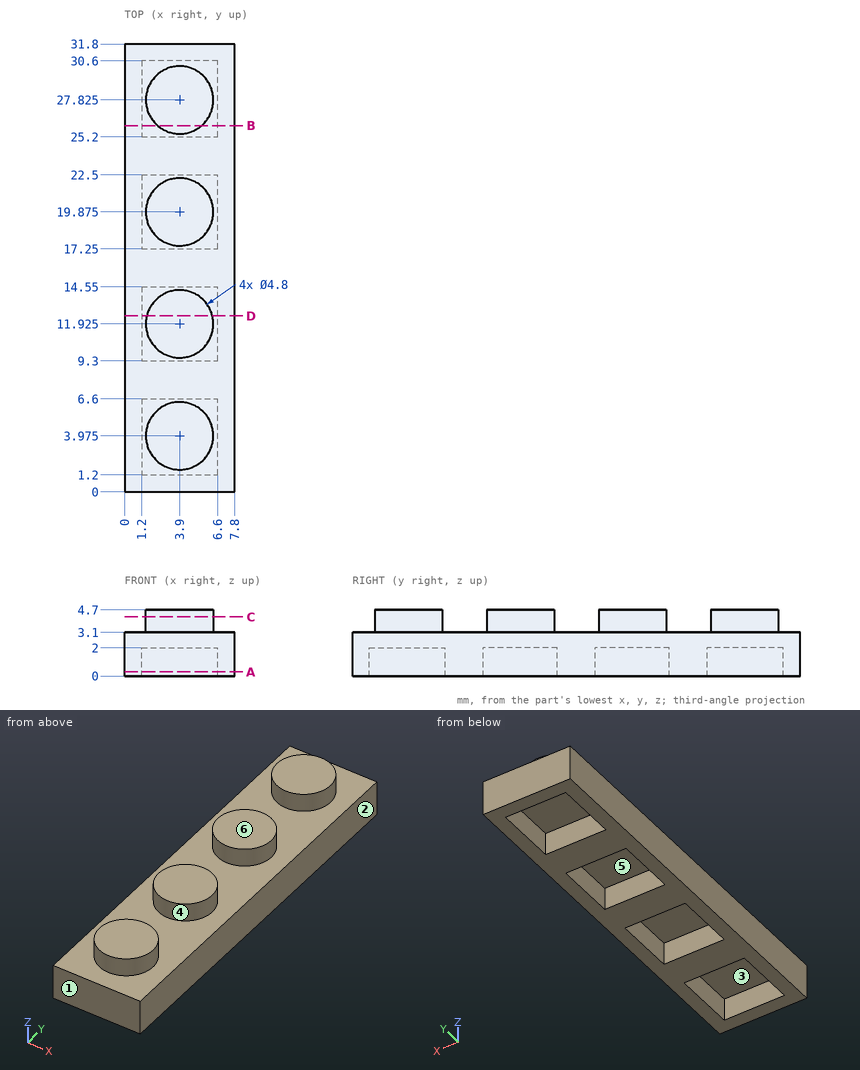
The figure shows three views and two pictorial views of one solid part (mm, origin at its lowest corner). Answer the questions. A direction names the side the tool comes from. Round coordinates to 2 decimals unless told otherwise and drop trailing zeros. Order: outer loops, then holes, each group sorted by start corner. A loop starts at its lowest first (then second) coordinate and runs counter-clockwise, first axis right, second up.
Q1. A cutting plane is placed at C-C, the plane z = 4.2. Determine the outline of the cut face in (x, y) (3 decimals), then the cut area to 3 significant figures.
Solution:
outline: circle Ø4.8 at (3.9, 3.975); circle Ø4.8 at (3.9, 11.925); circle Ø4.8 at (3.9, 19.875); circle Ø4.8 at (3.9, 27.825)
area: 72.4 mm2
Q2. A cutting plane is placed at A-A, the plane z = 0.3. Determine the outline of the cut face in (x, y).
Solution:
outline: (0, 0) - (7.8, 0) - (7.8, 31.8) - (0, 31.8) - close; hole (1.2, 1.2) - (6.6, 1.2) - (6.6, 6.6) - (1.2, 6.6) - close; hole (1.2, 9.3) - (6.6, 9.3) - (6.6, 14.55) - (1.2, 14.55) - close; hole (1.2, 17.25) - (6.6, 17.25) - (6.6, 22.5) - (1.2, 22.5) - close; hole (1.2, 25.2) - (6.6, 25.2) - (6.6, 30.6) - (1.2, 30.6) - close
Q3. Find the intervals of material crossed by line 1 along Y through (x, z) = (4.5, 1.8); line 2 along X through (y, z) = (9.5, 0.8); line 3 along Y through (x, z) = (1.75, 4.3), in increasing order.
Solution:
line 1: y = 0 to 1.2, 6.6 to 9.3, 14.55 to 17.25, 22.5 to 25.2, 30.6 to 31.8
line 2: x = 0 to 1.2, 6.6 to 7.8
line 3: y = 2.91 to 5.04, 10.86 to 12.99, 18.81 to 20.94, 26.76 to 28.89
Q4. Given pin 1 Ø2.5 at (x, y) = (3, 19) entering from -Z, flat-ended and moving along its own axis, determine where the tip first touches the part or whether it passes through.
Solution:
pin 1: stops at z = 2
Q5. The mould has two halves that part along Y. Classify the marked faces 1, 2 and 3: pulls with the +Y half, pulls with the -Y half, needs draft (parallel to the pull), parting line crosses it, or undercut.
Solution:
face 1: pulls with the -Y half
face 2: needs draft
face 3: undercut
Q6. A cutting plane is placed at B-B, the plane y = 26. Determine the outline of the cut face in (x, z), then the cut area to 3 significant figures.
Solution:
outline: (0, 0) - (1.2, 0) - (1.2, 2) - (6.6, 2) - (6.6, 0) - (7.8, 0) - (7.8, 3.1) - (5.46, 3.1) - (5.46, 4.7) - (2.34, 4.7) - (2.34, 3.1) - (0, 3.1) - close
area: 18.4 mm2
Q7. A cutting plane is placed at D-D, the plane y = 12.5. Determine the outline of the cut face in (x, z), then the cut area to 3 significant figures.
Solution:
outline: (0, 0) - (1.2, 0) - (1.2, 2) - (6.6, 2) - (6.6, 0) - (7.8, 0) - (7.8, 3.1) - (6.23, 3.1) - (6.23, 4.7) - (1.57, 4.7) - (1.57, 3.1) - (0, 3.1) - close
area: 20.8 mm2
Q8. A tool of negligible diameter and unlimited length cuts with its end or side. For the marked faces 4, 5 and 6, from which of +Z, -Z, +X, -X, +Y, -Y can it reach the whole face along a straight path? Write none if from no direction.
Solution:
face 4: +Z
face 5: -Z
face 6: +Z, +X, -X, +Y, -Y
